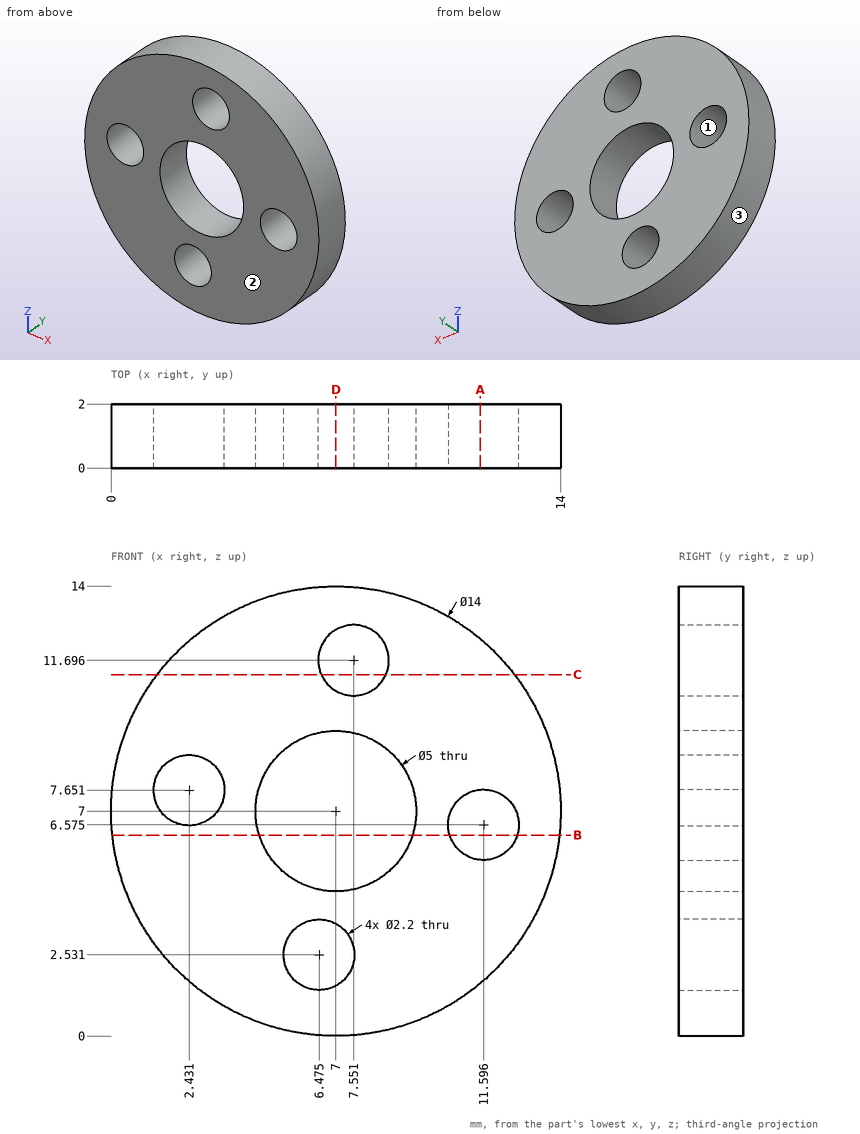
Study the drawing (mm; zero at the part's minimum x, y, z) and answer. Give positions to 0.01 mm unless a question says otherwise; leave off trailing zeros. Order: outer loops, then holes, each group sorted by start corner. A loop starts at its lowest first (then second) coordinate and runs counter-clockwise, first axis right, second up. Notation, with made-up numbers: M -6.75,52 L 44.25,52 A27 ccw 44.25,68 Z; hole C 56,43 d1. An arc over 180 degrees is marked long. Put each result on its own line as item: value. Start each with the question number.
Item 1: Flat-ended cylindrical pins translate along their axes: P1, Ø1, axis at y = 0.5, z = 2.5, coming from the +X side (1 decimal); P2, Ø1, axis at x = 12, y = 1.5, coming from the +Z side; P3, Ø1, axis at x = 9.5, y = 0.5, coming from the +Z side. Find the tip coordinate at first contact, or state that the pin passes through.
Item 2: The part is cut by section D-D, the plane x = 7. Determine the outline of the cut face in (y, z), and give its area (3 significant figures).
Item 3: Find the intervals of material crossed by line 1 along Z through (x, y) = (8.25, 0.95) (1 decimal); line 2 along X through (y, z) = (0.4, 6.25) (1 decimal); line 3 along Z through (x, y) = (5.25, 0.6) (1 decimal), in increasing order.
Item 4: The part is cut by section C-C, the plane z = 11.25. Determine the outline of the cut face in (x, y) (1 decimal).
Item 5: For a pull along X with two mould halves and no side action, classify the marked faces 1, 2 and 3 as +X half, -X half, draft (parallel to the pull), parting line (faces both ways), or undercut.
Item 6: The part is cut by section B-B, the plane z = 6.25. Determine the outline of the cut face in (x, y) (1 decimal).
Item 7: The part is cut by section A-A, the plane x = 11.5. Determine the outline of the cut face in (y, z).
Answer key:
1. P1: stops at x = 12.7
1. P2: stops at z = 12.36
1. P3: stops at z = 13.71
2. outline: M 0,0 L 2,0 L 2,1.56 L 0,1.56 Z; M 0,3.5 L 2,3.5 L 2,4.5 L 0,4.5 Z; M 0,9.5 L 2,9.5 L 2,10.74 L 0,10.74 Z; M 0,12.65 L 2,12.65 L 2,14 L 0,14 Z
2. area: 10.3 mm²
3. line 1: z = 0.1 to 4.8, 9.2 to 10.8, 12.5 to 13.9
3. line 2: x = 0 to 4.6, 9.4 to 10.5, 12.6 to 14
3. line 3: z = 0.2 to 5.2, 8.8 to 13.8
4. outline: M 1.4,0 L 6.5,0 L 6.5,2 L 1.4,2 Z; M 8.6,0 L 12.6,0 L 12.6,2 L 8.6,2 Z
5. face 1: undercut
5. face 2: draft
5. face 3: parting line
6. outline: M 0,0 L 4.6,0 L 4.6,2 L 0,2 Z; M 9.4,0 L 10.5,0 L 10.5,2 L 9.4,2 Z; M 12.6,0 L 14,0 L 14,2 L 12.6,2 Z
7. outline: M 0,1.64 L 2,1.64 L 2,5.48 L 0,5.48 Z; M 0,7.67 L 2,7.67 L 2,12.36 L 0,12.36 Z
